The drawing under review shows one solid part. Ordinate dimensions are in mm from its lowest x, y, z. A direction names the side the tool comes from. Give positions to 0.01 mm unless a question says otherwise; leave off trailing zeros. Write each loop counter-clockwise with the first axis right and the second up, starting at its lowest first coordinate (ties: lowest second). Pieces come first, ordered by that corner, then holes. Notation, with made-up numbers: (-1.75, 31) -> (2.25, 31) arc R27 cw to (2.25, 52) -> close; hole circle Ø6 at (-11, 30). An arc over 180 degrees is marked (long way). Answer as a JSON object with one key per item and string values.
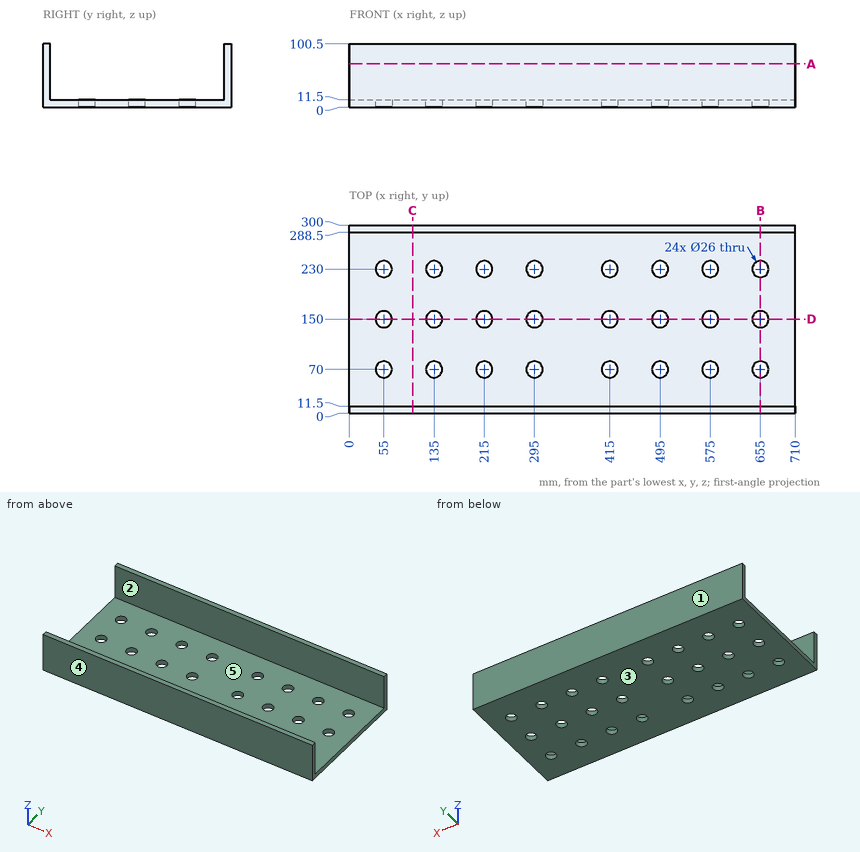
(1) We need section D-D, the plane y = 150. Give the number of separate pieces and of enclosed holes in the cut face, then the cut area to 3 significant figures.
Here are the results:
{"separate pieces": "9", "enclosed holes": "0", "area": "5,770 mm²"}
(2) We need section C-C, the plane x = 101. State the section outline as (y, z) points, then the cut area to 3 significant figures.
Here are the results:
{"outline": "(0, 0) -> (300, 0) -> (300, 100.5) -> (288.5, 100.5) -> (288.5, 11.5) -> (11.5, 11.5) -> (11.5, 100.5) -> (0, 100.5) -> close", "area": "5,500 mm²"}
(3) Clearance check with flat-ended pins moving along their axes: pin 1 (6 mm diameter, centred on x = 326.5, z = 59.5, fed in from -Y); pin 2 (10 mm diameter, centred on x = 213.5, y = 206.5, fed in from +Z). State where each tip first meets the part, or that it passes through.
Here are the results:
{"pin 1": "stops at y = 0", "pin 2": "stops at z = 11.5"}
(4) For the marked faces 1 and 2, list the 3-axis set-ups (+Z, -Z, +X, -X, +Y, -Y) from which the entire face can be reached by the end or side of a thin tool; tool diameter is ignored.
Here are the results:
{"face 1": "+Z, -Z, +X, -X, +Y", "face 2": "+Z, +X, -X"}
(5) We need section A-A, the plane z = 69. State the section outline as (x, y) points.
Here are the results:
{"outline": "(0, 0) -> (710, 0) -> (710, 11.5) -> (0, 11.5) -> close; (0, 288.5) -> (710, 288.5) -> (710, 300) -> (0, 300) -> close"}
(6) The part is to be moulded in two halves that separate along Y. For the marked faces 3, 4 and 5, say which applies: +Y half, -Y half, draft (parallel to the pull), parting line (faces both ways), or undercut.
Here are the results:
{"face 3": "draft", "face 4": "-Y half", "face 5": "undercut"}
(7) For line 1 along Y through (x, z) = (495, 6.25); line 2 along Y through (x, z) = (490, 71.5); line 3 along Z through (x, y) = (269.5, 23.5), list the stretches that pass through material, from the lowest coordinate up.
Here are the results:
{"line 1": "y = 0 to 57, 83 to 137, 163 to 217, 243 to 300", "line 2": "y = 0 to 11.5, 288.5 to 300", "line 3": "z = 0 to 11.5"}
(8) We need section B-B, the plane x = 655. State the section outline as (y, z) points.
Here are the results:
{"outline": "(0, 0) -> (57, 0) -> (57, 11.5) -> (11.5, 11.5) -> (11.5, 100.5) -> (0, 100.5) -> close; (83, 0) -> (137, 0) -> (137, 11.5) -> (83, 11.5) -> close; (163, 0) -> (217, 0) -> (217, 11.5) -> (163, 11.5) -> close; (243, 0) -> (300, 0) -> (300, 100.5) -> (288.5, 100.5) -> (288.5, 11.5) -> (243, 11.5) -> close"}
